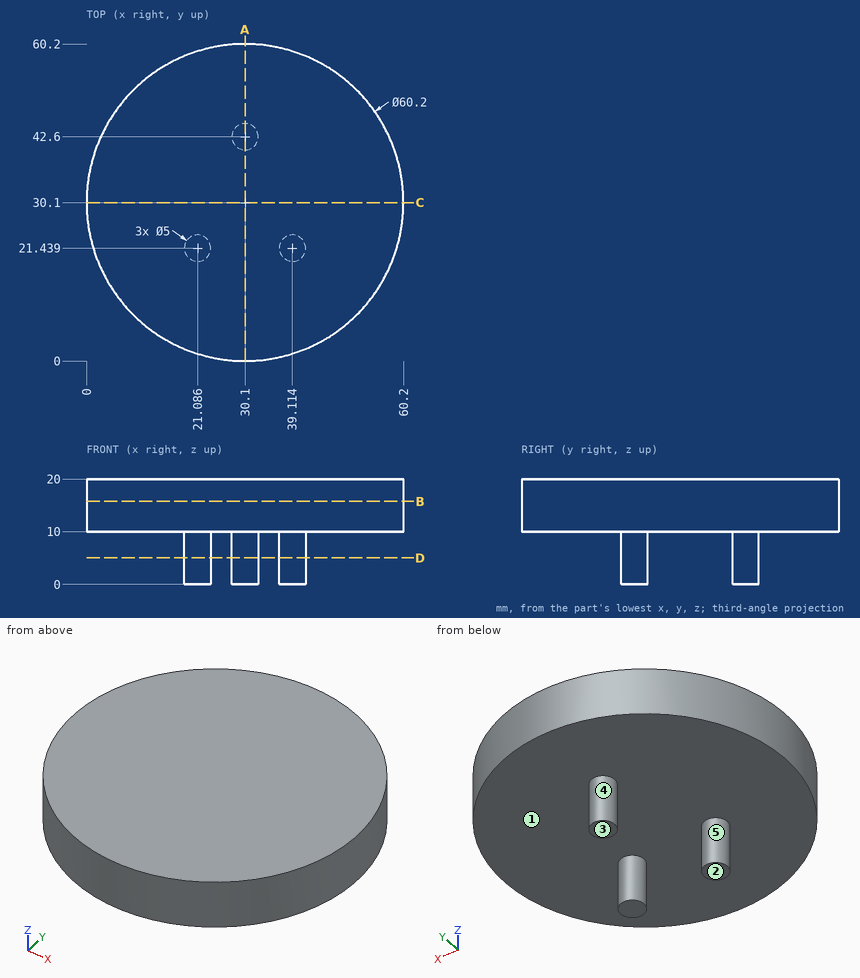
Verification items for this drawing (mm, ordinates from the low corner). A direction names the side the tool comes from. Coordinates: 2 decimals unless noted, no trailing zeros. Loops run counter-clockwise (first coordinate to the right, second up) from the corner with the lowest first, then second, coordinate; pieces in that order, holes last. Notation, with made-up numbers: (70, -36) - (118, -36) arc R12 ccw to (118, -14) - close; hole circle Ø11 at (67.25, -28.5). An arc over 180 degrees is marked (long way). One line per item, written item: value. Start each with the question number.
(1) Tool access check on the marked faces 1 and 2. Record the directions out of +Z, -Z, +X, -X, +Y, -Y that give a thin tool (end or side, any length) a straight path to the whole face; none if there is none.
(2) Mould release check, pull along X, two halves, no side actions. Record for the marked faces 3, 4 and 5: released by +X, released by -X, zero draft, split by the parting line, or undercut.
(3) Cross-section at B-B on z = 15.75. Enter the section's corners in (x, y).
(4) Depth check by flat-ended pin: P1, Ø1, axis at x = 25, z = 7, coming from the +Y side; P2, Ø8, axis at x = 13.5, y = 8.5, coming from the -Z side; P3, Ø2, axis at x = 31.5, z = 5, coming from the -Y side; P4, Ø18, axis at x = 22.5, y = 32, coming from the -Z side. Enter the tip coordinate at first touch or a pass-through.
(5) Cross-section at C-C on y = 30.1. Enter the section's corners in (x, z).
(6) Material ranges on line 1 (Z direction, x = 18, y = 24); line 2 (X direction, y = 20.5, z = 2.5); line 3 (X direction, y = 18, z = 17), recorded low to high. Write a range as [from, to].
(7) Cross-section at D-D on z = 5. Enter the section's corners in (x, y).
(8) Cross-section at A-A on x = 30.1. Enter the section's corners in (y, z), plus the area to 3 significant figures.
Results below:
1. face 1: -Z
1. face 2: -Z, +X, -X, +Y, -Y
2. face 3: zero draft
2. face 4: split by the parting line
2. face 5: undercut
3. outline: circle Ø60.2 at (30.1, 30.1)
4. P1: passes through
4. P2: stops at z = 10
4. P3: stops at y = 40.13
4. P4: stops at z = 0
5. outline: (0, 10) - (60.2, 10) - (60.2, 20) - (0, 20) - close
6. line 1: z = [10, 20]
6. line 2: x = [18.77, 23.4], [36.8, 41.43]
6. line 3: x = [2.54, 57.66]
7. outline: circle Ø5 at (21.09, 21.44); circle Ø5 at (30.1, 42.6); circle Ø5 at (39.11, 21.44)
8. outline: (0, 10) - (40.1, 10) - (40.1, 0) - (45.1, 0) - (45.1, 10) - (60.2, 10) - (60.2, 20) - (0, 20) - close
8. area: 652 mm2
